Geometry: final body of the model. Coordinates: model frame, mm. A direction names the side the tool comes from. Give positions to 0.01 mm unless a question says otherwise; leave off trailing zeros. Write each loop counter-clockwise with the first axis right and the second up, starting at its lowest first coordinate (ties: lowest second). Pieces come first, ordered by that corner, then holes.
Q1. Line query: line 1 (X direction, y = -8, z = 0); line 2 (X direction, y = 21, z = 0); line 3 (X direction, y = 19, z = 0). Output: solid intervals per line, ascending.
Q2. Pin query (flat end, axial travel): pin 1 Ø1.4 at (x, z) = (-11.5, -14) entering from -Y; pin 2 Ø8 at (x, y) = (0.5, -24.5) entering from -Z; pin 3 Ø1 at (y, z) = (-4.5, -3.5) entering from +X. Return the tip coordinate at first contact, or that it passes through.
Q3. Section B-B (x = 112.5). Return the cut outline in (y, z), plus the area to 3 significant figures.
Q4. Reachability of faces 1 (the flat face through (-10, 1.674, -14)), 2 (the flat face through (-2, 23.24, 25)), 3 (the cylindrical face through (7.304, -3.924, -0.2)), 4 (the flat face through (-10, -9, 12.7)), 5 (the flat face through (-10, 16.89, 0)) from +Z, -Z, +X, -X, +Y, -Y: full face, straight path, thin tool, end or side. Return the list, or none.
Q5. Section A-A (y = -16). Return the cut outline in (x, z), plus the area to 3 significant figures.
Q6. Mould query, pull axis Z, two halves, no side actions, for faces 6 (the cylindrical face through (-27.134, -14.797, 0.2)), 7 (the flat face through (152.4, -19, 0)), 8 (the flat face through (-10, -9, -12.7)), 9 (the cylindrical face through (15.27, 20.11, -3.31)). Classes: +Z half, -Z half, draft (parallel to the pull), parting line (faces both ways), or undercut.
Q7. Section C-C (y = -27). Return the cut outline in (x, z).
from build123d import *

# Parameters (mm, degrees)
BOSS_EXTRUDE1_DEPTH      = 50.8
BOSS_EXTRUDE1_DEPTH_BACK = 101.6
SKETCH2_R                = 12.7
CUT_EXTRUDE2_DEPTH       = 159.628919589
SKETCH4_R                = 25.4
CUT_EXTRUDE3_DEPTH       = 6.35


with BuildPart() as part:
    # Sketch1 → Revolve1 (revolve)
    with BuildSketch(Plane.XY, mode=Mode.PRIVATE) as revolve1_sk:
        with BuildLine():
            Line((28.184971871, 23.240239964), (-9.915028129, 23.240239964))
            Line((-9.915028129, 23.240239964), (-9.915028129, -36.426191716))
            Line((-9.915028129, -36.426191716), (7.305080495, -36.426191716))
            Line((7.305080495, -36.426191716), (7.305080495, 1.673808284))
            add(Edge.make_bspline(
                [(7.305080495, 1.673808284), (17.688890223, 5.05702424), (24.648854015, 12.2458348), (28.184971871, 23.240239964)],
                knots=[0.179471998, 0.179471998, 0.179471998, 0.179471998, 1, 1, 1, 1], degree=3))
        make_face()
    revolve(revolve1_sk.sketch.rotate(Axis((-9.915028129, 23.240239964, 0), (0, -1, 0)), 90), axis=Axis((-9.915028129, 23.240239964, 0), (0, -1, 0)))

    # Sketch2 → Boss-Extrude1 (add, two sides: drawn at the far end of the back side and taken through both)
    with BuildSketch(Plane(origin=(101.6, 0, 0), x_dir=(0, 0, -1), z_dir=(1, 0, 0)).offset(-BOSS_EXTRUDE1_DEPTH_BACK)):
        with Locations(Location((0, -18.998368254, 0), (0, 0, 180))):
            Circle(SKETCH2_R)
    extrude(amount=BOSS_EXTRUDE1_DEPTH + BOSS_EXTRUDE1_DEPTH_BACK)

    # Sketch3 → Cut-Extrude2 (cut, through all)
    with BuildSketch(Plane(origin=(101.6, 0, 0), x_dir=(0, 0, -1), z_dir=(1, 0, 0))):
        with BuildLine():
            Line((17.220108624, -36.426191716), (17.220108624, -18.998368254))
            Line((17.220108624, -18.998368254), (17.220108624, 1.673808284))
            Line((17.220108624, 1.673808284), (12.7, 1.673808284))
            Line((12.7, 1.673808284), (12.7, -18.998368254))
            ThreePointArc((12.7, -18.998368254), (0, -31.698368254), (-12.7, -18.998368254))
            Line((-12.7, -18.998368254), (-12.7, 1.673808284))
            Line((-12.7, 1.673808284), (-17.220108624, 1.673808284))
            Line((-17.220108624, 1.673808284), (-17.220108624, -18.998368254))
            Line((-17.220108624, -18.998368254), (-17.220108624, -36.426191716))
            Line((-17.220108624, -36.426191716), (17.220108624, -36.426191716))
        make_face()
    extrude(amount=-CUT_EXTRUDE2_DEPTH, mode=Mode.SUBTRACT)

    # Sketch4 → Cut-Extrude3 (cut)
    with BuildSketch(Plane(origin=(0, 23.240239964, 0), x_dir=(1, 0, 0), z_dir=(0, 1, 0))):
        with Locations(Location((-9.915028129, 0, 0), (0, 0, 270))):
            Circle(SKETCH4_R)
    extrude(amount=-CUT_EXTRUDE3_DEPTH, mode=Mode.SUBTRACT)


solid = part.part
Computed:
1. line 1: x = -27.14 to 152.4
1. line 2: x = -47.23 to -35.32, 15.48 to 27.4
1. line 3: x = -46.4 to -35.32, 15.48 to 26.57
2. pin 1: stops at y = 1.67
2. pin 2: stops at z = -12.61
2. pin 3: stops at x = 7.04
3. outline: circle Ø25.4 at (-19, 0)
3. area: 507 mm2
4. face 1: -Z, +X, -X, -Y
4. face 2: +Z, -Z, +X, -X, +Y
4. face 3: +X
4. face 4: +Z, +X, -X, -Y
4. face 5: +Y
5. outline: (-21.54, -12.7) - (1.71, -12.7) arc R17.22 ccw to (2.09, -12.34) - (152.4, -12.34) - (152.4, 12.34) - (2.09, 12.34) arc R17.22 ccw to (1.71, 12.7) - (-21.54, 12.7) arc R17.22 ccw to start
5. area: 4,410 mm2
6. face 6: parting line
6. face 7: draft
6. face 8: -Z half
6. face 9: undercut
7. outline: (-24.03, -9.86) - (152.4, -9.86) - (152.4, 9.86) - (-24.03, 9.86) arc R17.22 ccw to start
